from build123d import *

# Parameters (mm, degrees)
BOSS_EXTRUDE1_DEPTH = 42
SKETCH2_W           = 0.75
SKETCH2_H           = 1.6
FILLET1_R           = 0.6


with BuildPart() as part:
    # Sketch1 → Boss-Extrude1 (new body)
    with BuildSketch(Plane.XY):
        with BuildLine():
            Line((-8, 13.856406461), (-7.15, 12.384163274))
            ThreePointArc((-7.15, 12.384163274), (0, -14.3), (7.15, 12.384163274))
            Line((7.15, 12.384163274), (7.986524529, 13.864177795))
            ThreePointArc((7.986524529, 13.864177795), (0.007777885, -15.99999811), (-8, 13.856406461))
        make_face()
    extrude(amount=BOSS_EXTRUDE1_DEPTH)

    # Sketch2 → Cut-Revolve1 (revolve, cut)
    with BuildSketch(Plane(origin=(0, 0, 0), x_dir=(1, 0, 0), z_dir=(0, 1, 0))):
        with Locations((15.625, -35.45)):
            Rectangle(SKETCH2_W, SKETCH2_H)
        with Locations((15.625, -6.55)):
            Rectangle(SKETCH2_W, SKETCH2_H)
    revolve(axis=Axis((0, 0, 0), (0, 0, 1)), mode=Mode.SUBTRACT)

    # Fillet1
    fillet1_edges = [part.edges().sort_by_distance(p)[0] for p in [
        (0.007777885, -15.99999811, 42),
        (0.007777885, -15.99999811, 0),
    ]]
    fillet(fillet1_edges, radius=FILLET1_R)


solid = part.part
Input: part model. Units: mm. Frame: model coordinates. A direction names the side the tool comes from. Coordinates: 2 decimals unless noted, no trailing zeros. Order: outer loops, then holes, each group sorted by start corner. A loop starts at its lowest first (then second) coordinate and runs counter-clockwise, first axis right, second up.
1. Access query for faces 5 (the flat face through (0.1, -15.4, 34.65)), 6 (the flat face through (-7.58, 13.13, 20.71)), 7 (the cylindrical face through (-0.52, -14.29, 20.71)). Directions: +Z, -Z, +X, -X, +Y, -Y. A direction counts if a zero-diameter tool reaches every point of the face in a straight line with its end or side. Return the directions, or none.
Checked values:
face 5: none
face 6: +Z, -Z, +Y
face 7: +Z, -Z
2. Draft query along Z for faces 1 (the cylindrical face through (0.59, -15.99, 3.14)), 2 (the flat face through (0.1, -15.4, 36.25)), 3 (the flat face through (0.1, -15.4, 5.75)), 4 (the flat face through (5, -14, 0)). Return one class per face: +Z half, -Z half, draft (parallel to the pull), parting line (faces both ways), or undercut.
Checked values:
face 1: draft
face 2: undercut
face 3: undercut
face 4: -Z half
3. Contact query for flat-ended pins moving along their axis: P1, Ø3, axis at x = -7.5, z = 22, coming from the -Y side; P2, Ø8, axis at x = -11.5, z = 7.5, coming from the +Y side; P3, Ø10, axis at y = -6.5, z = 32.5, coming from the -X side. Output: stop coordinate, or through.
Checked values:
P1: stops at y = -14.83
P2: stops at y = 13.86
P3: stops at x = -15.93
4. Cut plane A-A, the plane z = 25.5. Return loops of the section in (x, y).
Checked values:
outline: (-8, 13.86) arc R16 ccw (long way) to (7.99, 13.86) - (7.15, 12.38) arc R14.3 cw (long way) to (-7.15, 12.38) - close
5. Ray query, line 1 along X through (y, z) = (0.5, 37.5); line 2 along Y through (x, z) = (0, 9); line 3 along X through (y, z) = (7.5, 29). Return the intervals inside material, ascending.
Checked values:
line 1: x = -15.99 to -14.29, 14.29 to 15.99
line 2: y = -16 to -14.3
line 3: x = -14.13 to -12.18, 12.18 to 14.13
